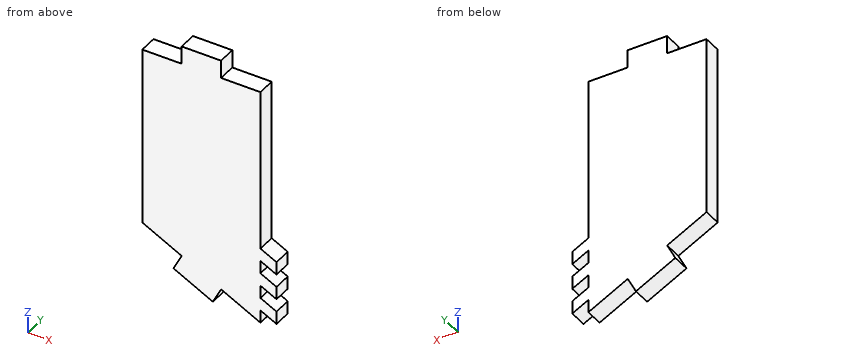
```python
from build123d import *

# Parameters (mm, degrees)
BOSS_EXTRUDE1_DEPTH = 3
SKETCH2_W           = 6.55
SKETCH2_H           = 3
BOSS_EXTRUDE2_DEPTH = 3


with BuildPart() as part:
    # Sketch1 → Boss-Extrude1 (new body)
    with BuildSketch(Plane(origin=(0, 0, 0), x_dir=(1, 0, 0), z_dir=(0, 1, 0))):
        Polygon((0, 30), (19.65, 40), (19.65, 30), (19.65, 0), (0, 0), align=None)
    extrude(amount=BOSS_EXTRUDE1_DEPTH)

    # Sketch2 → Boss-Extrude2 (add)
    with BuildSketch(Plane.XZ):
        Polygon((13.099461063, -36.666392399), (11.7388049, -39.340081761), (5.188265963, -36.006474159), (6.548922127, -33.332784797), align=None)
        Polygon((19.65, -27.142857143), (22.323732333, -28.503428866), (22.323732333, -30.646285866), (19.65, -29.285714143), align=None)
        Polygon((19.65, -31.428571143), (22.323732333, -32.789142866), (22.323732333, -34.931999866), (19.65, -33.571428143), align=None)
        Polygon((19.65, -35.714285143), (22.323732333, -37.074856866), (22.323732333, -39.217713866), (19.65, -37.857142143), align=None)
        with Locations((9.825, 1.5)):
            Rectangle(SKETCH2_W, SKETCH2_H)
    extrude(amount=-BOSS_EXTRUDE2_DEPTH)


solid = part.part
```
Geometry check sheet. Reference: the model listing, model coordinates, mm. Coordinates: 2 decimals unless noted, no trailing zeros. Order: outer loops, then holes, each group sorted by start corner. A loop starts at its lowest first (then second) coordinate and runs counter-clockwise, first axis right, second up.
Q1. Depth check by flat-ended pin: pin 1 Ø0.9 at (y, z) = (1, -19) entering from +X; pin 2 Ø1.5 at (y, z) = (0.5, -2) entering from -X; pin 3 Ø1.5 at (x, y) = (17.5, 1.5) entering from +Z. Enter the tip coordinate at first touch or a pass-through.
Reply:
pin 1: stops at x = 19.65
pin 2: stops at x = 0
pin 3: stops at z = 0
Q2. Thickness scan on probe 1 along Z at (x, y) = (20.75, 2.75); probe 2 along Z at (x, y) = (20, 0.6); probe 3 along X at (y, z) = (0.4, -13). Record the ranges inside material, lowest first.
Reply:
probe 1: z = -38.42 to -36.27, -34.13 to -31.99, -29.85 to -27.7
probe 2: z = -38.04 to -35.89, -33.75 to -31.61, -29.46 to -27.32
probe 3: x = 0 to 19.65
Q3. Sectioned sample at D-D on x = 4. Record the cut outline in (y, z), and give its area (3 significant figures).
Reply:
outline: (0, -32.04) - (3, -32.04) - (3, 0) - (0, 0) - close
area: 96.1 mm2
Q4. Sectioned sample at C-C on z = -18. Record the cut outline in (x, y), and give its area (4 significant figures).
Reply:
outline: (0, 0) - (19.65, 0) - (19.65, 3) - (0, 3) - close
area: 58.95 mm2
Q5. Sectioned sample at B-B on y = 1. Record the cut outline in (x, z).
Reply:
outline: (0, -30) - (6.55, -33.33) - (5.19, -36.01) - (11.74, -39.34) - (13.1, -36.67) - (19.65, -40) - (19.65, -37.86) - (22.32, -39.22) - (22.32, -37.07) - (19.65, -35.71) - (19.65, -33.57) - (22.32, -34.93) - (22.32, -32.79) - (19.65, -31.43) - (19.65, -29.29) - (22.32, -30.65) - (22.32, -28.5) - (19.65, -27.14) - (19.65, 0) - (13.1, 0) - (13.1, 3) - (6.55, 3) - (6.55, 0) - (0, 0) - close
Q6. Sectioned sample at A-A on x = 20.25. Record the cut outline in (y, z), and give its area (3 significant figures).
Reply:
outline: (0, -38.16) - (3, -38.16) - (3, -36.02) - (0, -36.02) - close; (0, -33.88) - (3, -33.88) - (3, -31.73) - (0, -31.73) - close; (0, -29.59) - (3, -29.59) - (3, -27.45) - (0, -27.45) - close
area: 19.3 mm2
